from build123d import *

# Parameters (mm, degrees)
F0_W     = 381
F0_H     = 1281.049
F1_DEPTH = 5.334
F3_DEPTH = 25.4
F4_W     = 381
F4_H     = 44.45
F5_DEPTH = 25.4
F6_R     = 4.7625
F7_DEPTH = 25.4


with BuildPart() as f1:
    # F0 (on Front) → F1 (new body)
    with BuildSketch(Plane.XZ):
        with Locations((-304.8, 640.5245)):
            Rectangle(F0_W, F0_H)
    extrude(amount=F1_DEPTH)

    # F2 (on face) → F3 (cut)
    with BuildSketch(Plane.XZ.offset(5.334)):
        with BuildLine():
            Line((-114.3, 1103.249), (-114.3, 1281.049))
            Line((-114.3, 1281.049), (-215.9, 1281.049))
            Line((-215.9, 1281.049), (-215.9, 1115.949))
            ThreePointArc((-215.9, 1115.949), (-212.180256, 1106.968744), (-203.2, 1103.249))
            Line((-203.2, 1103.249), (-114.3, 1103.249))
        make_face()
    extrude(amount=-F3_DEPTH, mode=Mode.SUBTRACT)

    # F4 (on face) → F5 (cut)
    with BuildSketch(Plane.XZ.offset(5.334)):
        with Locations((-304.8, 22.225)):
            Rectangle(F4_W, F4_H)
    extrude(amount=-F5_DEPTH, mode=Mode.SUBTRACT)

    # F6 (on face) → F7 (cut)
    with BuildSketch(Plane.XZ.offset(5.334)):
        with Locations((-266.7, 1230.249)):
            Circle(F6_R)
    extrude(amount=-F7_DEPTH, mode=Mode.SUBTRACT)


solid = f1.part
Build history of the part. All positions in model axes, mm. Give positions to 0.01 mm unless a question says otherwise; leave off trailing zeros. Order: outer loops, then holes, each group sorted by start corner. A loop starts at its lowest first (then second) coordinate and runs counter-clockwise, first axis right, second up. Notation, with made-up numbers: M -1,-27.75 L 27,-27.75 A23 ccw 27,9.25 Z; hole C 41.25,-9.75 d4. An arc over 180 degrees is marked long. Put each result on its own line as item: value.
Item 1: Slice it at B-B, the plane x = -156.5. Write the cut outline in (y, z).
From the geometry:
outline: M -5.33,44.45 L 0,44.45 L 0,1103.25 L -5.33,1103.25 Z
Item 2: Flat gauge pins, fed straight in: pin 1 Ø1.6 at (y, z) = (-3.5, 1220) entering from +X; pin 2 Ø2.5 at (x, y) = (-177, -1.5) entering from +Z. Where does each tip first touch, or does it go through?
From the geometry:
pin 1: stops at x = -215.9
pin 2: stops at z = 1103.25
Item 3: Probe line 1 (Z direction, x = -266.7, y = -1.3); line 2 (Z direction, x = -156, y = -3.45); line 3 (X direction, y = -1, z = 1151). List the from-to ranges inside material, lowest first. Write a range as [from, to].
From the geometry:
line 1: z = [44.45, 1225.49], [1235.01, 1281.05]
line 2: z = [44.45, 1103.25]
line 3: x = [-495.3, -215.9]
